Geometry check sheet. Reference: the model listing, model coordinates, mm. Face numbers are marked on the shaded views. A direction names the side the tool comes from. Coordinates: 2 decimals unless noted, no trailing zeros. Write each loop counter-clockwise with the first axis right and the second up, starting at its lowest first coordinate (ties: lowest second). Pieces come first, ordered by that corner, then holes. Notation, with made-up numbers: M 1,4 L 7,4 A20 ccw 7,29 Z; hole C 44,-34.75 d8. An arc over 180 degrees is marked long. Write item = value, one per line. Start each with the question number.
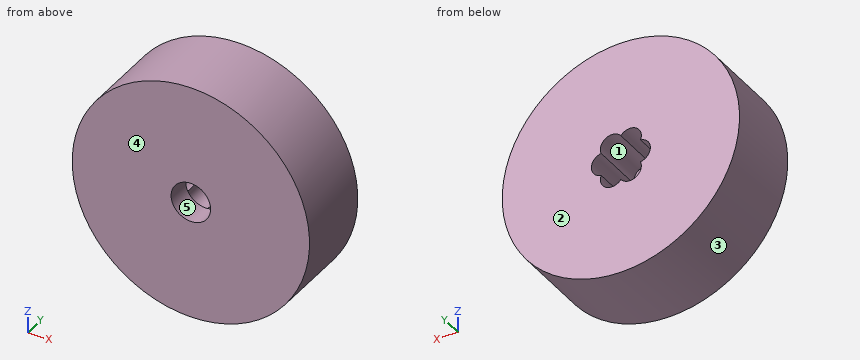
```python
from build123d import *

# Parameters (mm, degrees)
SKETCH1_R           = 30
BOSS_EXTRUDE1_DEPTH = 20
SKETCH2_R           = 5
CUT_EXTRUDE1_DEPTH  = 47.904157598
SKETCH3_R           = 2.898603643
CUT_EXTRUDE2_DEPTH  = 13.9375
CIRPATTERN1_START   = 6.062499991
CIRPATTERN1_DEPTH   = 13.937500009


# Read off the part's stored shape, not the designer's step: CirPattern1
with BuildPart() as part:
    # Sketch1 → Boss-Extrude1 (new body)
    with BuildSketch(Plane(origin=(0, 0, 0), x_dir=(1, 0, 0), z_dir=(0, 1, 0))):
        with Locations(Location((0, 0, 0), (0, 0, 270))):
            Circle(SKETCH1_R)
    extrude(amount=BOSS_EXTRUDE1_DEPTH)

    # Sketch2 → Cut-Extrude1 (cut, through all)
    with BuildSketch(Plane(origin=(0, 0, 0), x_dir=(1, 0, 0), z_dir=(0, 1, 0))):
        with Locations(Location((0, 0, 0), (0, 0, 270))):
            Circle(SKETCH2_R)
    extrude(amount=CUT_EXTRUDE1_DEPTH, mode=Mode.SUBTRACT)

    # Sketch3 → Cut-Extrude2 (cut)
    with BuildSketch(Plane(origin=(0, 20, 0), x_dir=(1, 0, 0), z_dir=(0, 1, 0))):
        with Locations((-4.564381882, 0)):
            Circle(SKETCH3_R)
    extrude(amount=-CUT_EXTRUDE2_DEPTH, mode=Mode.SUBTRACT)

    # CirPattern1 outline → CirPattern1 (cut)
    with BuildSketch(Plane(origin=(0, 0, 0), x_dir=(1, 0, 0), z_dir=(0, 1, 0)).offset(CIRPATTERN1_START)):
        with BuildLine():
            ThreePointArc((-4.10041051, -2.861229394), (-4.535329521, -2.898458045), (-4.970907389, -2.869954719))
            ThreePointArc((-4.970907389, -2.869954719), (-3.731492762, -6.463135052), (0, -5.739909439))
            ThreePointArc((0, -5.739909439), (3.731492762, -6.463135052), (4.970907389, -2.869954719))
            ThreePointArc((4.970907389, -2.869954719), (7.462985525, 0), (4.970907389, 2.869954719))
            ThreePointArc((4.970907389, 2.869954719), (3.731492762, 6.463135052), (0, 5.739909439))
            ThreePointArc((0, 5.739909439), (-3.731492762, 6.463135052), (-4.970907389, 2.869954719))
            ThreePointArc((-4.970907389, 2.869954719), (-4.535329521, 2.898458045), (-4.10041051, 2.861229394))
            ThreePointArc((-4.10041051, 2.861229394), (5, 0), (-4.10041051, -2.861229394))
        make_face()
    extrude(amount=CIRPATTERN1_DEPTH, mode=Mode.SUBTRACT)


solid = part.part
```
Q1. Cross-section at D-D on z = -21. Enter the section's corners in (x, y), and give its area (3 significant figures).
Q2. Cross-section at C-C on y = 2.25. Enter the section's corners in (x, z), and give its area (3 significant figures).
Q3. Cross-section at A-A on z = 0. Enter the section's corners in (x, y).
Q4. Set-up check for the marked faces 1 and 2: record each of +Z, -Z, +X, -X, +Y, -Y from which the full face is reachable in a straight line by a thin tool's end or side.
Q5. Cross-section at B-B on x = -24. Enter the section's corners in (y, z), and give its area (3 significant figures).
Q6. Gauge pin test, flat ends, axial feed: pin 1 (12 mm diameter, centred on y = 7, z = -15.5, fed in from -X); pin 2 (15 mm diameter, centred on x = 3, z = 0.5, fed in from +Y); pin 3 (5 mm diameter, centred on y = 10, z = 13.5, fed in from -X); pin 4 (3 mm diameter, centred on y = 15, z = -12, fed in from -X). Record the tip position at first contact, or that the pin passes through.
Q7. Draft check along X on the marked faces 3, 4 and 5. Enter one of: pulls with the +X half, pulls with the -X half, needs draft (parallel to the pull), parting line crosses it, or undercut.
Q8. Scan lines: L1, parallel to X at y = 2, z = 0; L2, parallel to X at y = 2, z = 3; L3, parallel to Z at x = 1, y = 3.75. Record each from-to range of solid material in increasing order.
Values found:
q1.outline = M -21.42,0 L 21.42,0 L 21.42,20 L -21.42,20 Z
q1.area = 857 mm²
q2.outline = C 0,0 d60; hole C 0,0 d10
q2.area = 2,750 mm²
q3.outline = M -30,0 L -5,0 L -5,6.06 L -7.46,6.06 L -7.46,20 L -30,20 Z; M 5,0 L 30,0 L 30,20 L 7.46,20 L 7.46,6.06 L 5,6.06 Z
q4.face_1 = +Y
q4.face_2 = +Z, -Z, +X, -X, +Y
q5.outline = M 0,-18 L 20,-18 L 20,18 L 0,18 Z
q5.area = 720 mm²
q6.pin_1 = -28.46
q6.pin_2 = 20
q6.pin_3 = -27.91
q6.pin_4 = -28.1
q7.face_3 = parting line crosses it
q7.face_4 = needs draft
q7.face_5 = undercut
q8.L1 = -30 to -5, 5 to 30
q8.L2 = -29.85 to -4, 4 to 29.85
q8.L3 = -29.98 to -4.9, 4.9 to 29.98
